Geometry check sheet. Reference: the model listing, model coordinates, mm. A direction names the side the tool comes from. Round coordinates to 2 decimals unless told otherwise and drop trailing zeros. Order: outer loops, then holes, each group sorted by start corner. A loop starts at its lowest first (then second) coordinate and runs counter-clockwise, first axis right, second up.
(1) Sectioned sample at C-C (x = 2.55). Give the number of separate pieces and of enclosed holes in the cut face, plus the area to 3 significant figures.
(2) Material ranges on line 1 along Y through (x, z) = (2.9, -44); line 2 along Z through (x, y) = (2.25, 18.5) (3 decimals); line 3 along Y through (x, z) = (2.85, 84), recorded low to high.
(3) Go/stop test with flat-tipped pins: pin 1 (1 mm diameter, centred on x = 2, z = 112.5, fed in from +Y); pin 2 (1 mm diameter, centred on x = 1, y = 20, fed in from -Z) (3 decimals); pin 3 (1.5 mm diameter, centred on x = 1, y = 14, fed in from -Z). Record where each tip stops, or that it passes through.
(4) Sectioned sample at D-D (z = 67.5). Record the boundary of the cut face in (x, y) (3 decimals), plus the area to 4 significant figures.
(5) Release check for a two-part mould opening along Z. For faces 1 (the face through (1.57, 13.87, -102.44)), 2 (the face through (1.57, 6.37, -20.82)), 3 (the face through (1.6, 34.1, -82.1)) record: +Z half, -Z half, draft (parallel to the pull), parting line (faces both ways), or undercut.
(6) Set-up check for faces 4 (the face through (1.565, -30.21, 94.895)), 5 (the face through (1.57, 23.97, 95.82)), 6 (the face through (1.57, 6.43, -98.63)): record each of +Z, -Z, +X, -X, +Y, -Y from which the full face is reachable in a straight line by a thin tool's end or side.
(7) Sectioned sample at B-B (y = 0). Record the boundary of the cut face in (x, z) (3 decimals).
(8) Sectioned sample at A-A (z = -41.5). Record the boundary of the cut face in (x, y) (3 decimals), plus the area to 3 significant figures.
from build123d import *

# Parameters (mm, degrees)
SKETCH1_R           = 7.5
BOSS_EXTRUDE1_DEPTH = 3.175


with BuildPart() as part:
    # Sketch1 → Boss-Extrude1 (new body)
    with BuildSketch(Plane(origin=(0, 0, 0), x_dir=(0, 0, -1), z_dir=(1, 0, 0))):
        with BuildLine():
            Line((-94.755, 15), (-94.755, 18.175))
            Line((-94.755, 18.175), (-97.93, 18.175))
            Line((-97.93, 18.175), (-97.93, 21.35))
            Line((-97.93, 21.35), (-94.755, 21.35))
            ThreePointArc((-94.755, 21.35), (-95.853349571, 24.001650429), (-98.505, 25.1))
            Line((-98.505, 25.1), (-106.005, 25.1))
            ThreePointArc((-106.005, 25.1), (-108.656650429, 24.001650429), (-109.755, 21.35))
            Line((-109.755, 21.35), (-106.58, 21.35))
            Line((-106.58, 21.35), (-106.58, 18.175))
            Line((-106.58, 18.175), (-109.755, 18.175))
            Line((-109.755, 18.175), (-109.755, 15))
            Line((-109.755, 15), (-117.255, 15))
            ThreePointArc((-117.255, 15), (-119.022766953, 14.267766953), (-119.755, 12.5))
            Line((-119.755, 12.5), (-119.755, 7.5))
            ThreePointArc((-119.755, 7.5), (-119.022766953, 5.732233047), (-117.255, 5))
            Line((-117.255, 5), (-109.755, 5))
            Line((-109.755, 5), (-109.755, -12))
            Line((-109.755, -12), (-114.755, -12))
            Line((-114.755, -12), (-114.755, -13.5))
            Line((-114.755, -13.5), (-117.255, -13.5))
            Line((-117.255, -13.5), (-117.255, -12))
            ThreePointArc((-117.255, -12), (-119.755, -14.5), (-117.255, -17))
            Line((-117.255, -17), (-109.755, -17))
            Line((-109.755, -17), (-109.755, -27))
            Line((-109.755, -27), (-117.255, -27))
            ThreePointArc((-117.255, -27), (-119.022766953, -27.732233047), (-119.755, -29.5))
            Line((-119.755, -29.5), (-119.755, -37.5))
            ThreePointArc((-119.755, -37.5), (-119.022766953, -39.267766953), (-117.255, -40))
            Line((-117.255, -40), (-117.255, -36.825))
            Line((-117.255, -36.825), (-114.755, -36.825))
            Line((-114.755, -36.825), (-114.755, -40))
            Line((-114.755, -40), (-109.755, -40))
            Line((-109.755, -40), (-109.755, -45))
            Line((-109.755, -45), (-104.755, -45))
            Line((-104.755, -45), (-84.755, -15))
            Line((-84.755, -15), (99.755, -15))
            ThreePointArc((99.755, -15), (102.406650429, -13.901650429), (103.505, -11.25))
            Line((103.505, -11.25), (103.505, 11.25))
            ThreePointArc((103.505, 11.25), (102.406650429, 13.901650429), (99.755, 15))
            Line((99.755, 15), (96.005, 15))
            Line((96.005, 15), (96.005, 28.275))
            Line((96.005, 28.275), (92.83, 28.275))
            Line((92.83, 28.275), (92.83, 31.45))
            Line((92.83, 31.45), (96.005, 31.45))
            ThreePointArc((96.005, 31.45), (94.906650429, 34.101650429), (92.255, 35.2))
            Line((92.255, 35.2), (84.755, 35.2))
            ThreePointArc((84.755, 35.2), (82.103349571, 34.101650429), (81.005, 31.45))
            Line((81.005, 31.45), (84.18, 31.45))
            Line((84.18, 31.45), (84.18, 28.275))
            Line((84.18, 28.275), (81.005, 28.275))
            Line((81.005, 28.275), (81.005, 15))
            Line((81.005, 15), (-94.755, 15))
        make_face()
        with Locations((-92.255, 0)):
            Circle(SKETCH1_R, mode=Mode.SUBTRACT)
        with BuildLine():
            Line((23.505, 7.5), (96.005, 7.5))
            ThreePointArc((96.005, 7.5), (98.656650429, 6.401650429), (99.755, 3.75))
            Line((99.755, 3.75), (99.755, -3.75))
            ThreePointArc((99.755, -3.75), (98.656650429, -6.401650429), (96.005, -7.5))
            Line((96.005, -7.5), (23.505, -7.5))
            ThreePointArc((23.505, -7.5), (20.853349571, -6.401650429), (19.755, -3.75))
            Line((19.755, -3.75), (19.755, 3.75))
            ThreePointArc((19.755, 3.75), (20.853349571, 6.401650429), (23.505, 7.5))
        make_face(mode=Mode.SUBTRACT)
    extrude(amount=BOSS_EXTRUDE1_DEPTH)


solid = part.part
Answer below:
1. separate pieces: 1
1. enclosed holes: 2
1. area: 6,140 mm2
2. line 1: y = -15 to -7.5, 7.5 to 15
2. line 2: z = -96.005 to -81.005, 97.93 to 106.58
2. line 3: y = -15 to 15
3. pin 1: stops at y = 15
3. pin 2: stops at z = -96.005
3. pin 3: stops at z = -102.93
4. outline: (0, -15) - (3.175, -15) - (3.175, 15) - (0, 15) - close
4. area: 95.25 mm2
5. face 1: -Z half
5. face 2: undercut
5. face 3: +Z half
6. face 4: -Z, +X, -X, -Y
6. face 5: +X, -X, +Y
6. face 6: +X, -X
7. outline: (0, -103.505) - (3.175, -103.505) - (3.175, -99.755) - (0, -99.755) - close; (0, -19.755) - (3.175, -19.755) - (3.175, 84.755) - (0, 84.755) - close; (0, 99.755) - (3.175, 99.755) - (3.175, 109.755) - (0, 109.755) - close
8. outline: (0, -15) - (3.175, -15) - (3.175, -7.5) - (0, -7.5) - close; (0, 7.5) - (3.175, 7.5) - (3.175, 15) - (0, 15) - close
8. area: 47.6 mm2
